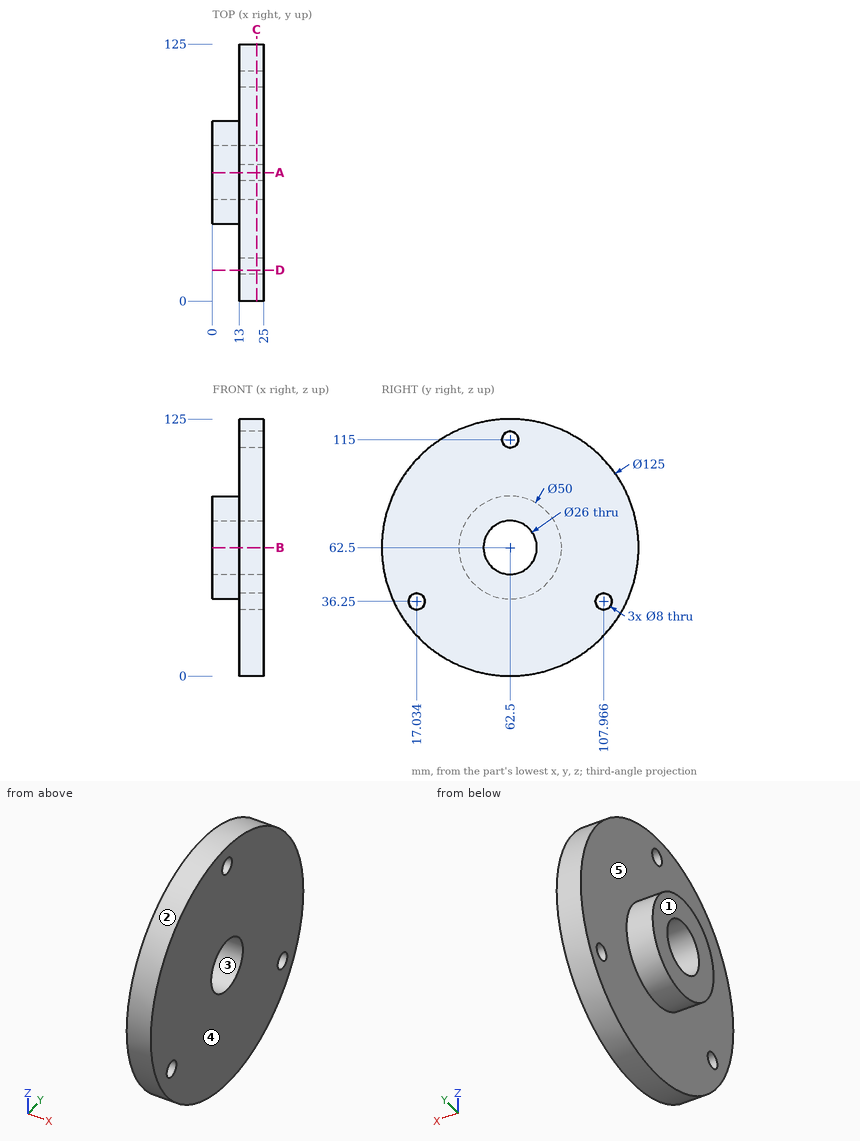
For this review, use the dimensioned drawing (mm, ordinates from the lowest corner) and the shaded views. A direction names the side the tool comes from. Give positions to 0.01 mm unless a question says otherwise; leave off trailing zeros. Loops run counter-clockwise (first coordinate to the right, second up) from the corner with the lowest first, then second, coordinate; pieces in that order, holes last.
Item 1: Tool access review of the marked faces 4 and 5: name each direction out of +Z, -Z, +X, -X, +Y, -Y from which nothing blocks a thin tool from reaching the whole face with its end or side.
Item 2: Insertion check: pin 1 (10.5 mm diameter, centred on y = 107.97, z = 36.25, fed in from +X); pin 2 (2 mm diameter, centred on x = 19.5, y = 81.5, fed in from +Z); pin 3 (10 mm diameter, centred on x = 10, y = 48.5, fed in from +Z) (1 decimal); pin 4 (1.5 mm diameter, centred on x = 6.5, z = 43, fed in from +Y) (1 decimal). Each pin has a flat end and moves straight along its axis. Give the tip position at first contact, or say it passes through.
Item 3: Take a section at A-A, the plane y = 62.5. State the section outline as (x, z) points, and give its area (3 significant figures).
Item 4: Take a section at C-C, the plane x = 21.5. State the section outline as (y, z) points.
Item 5: Take a section at D-D, the plane y = 15. State the section outline as (x, z) points (1 decimal).
Item 6: Take a section at B-B, the plane z = 62.5. State the section outline as (x, y) points.
Item 7: Draft analysis for pull direction Y (two halves, no side actions). For the marked faces 1, 2 and 3, state which applies: +Y half, -Y half, draft (parallel to the pull), parting line (faces both ways), or undercut.
Item 8: For line 1 along Y through (x, z) = (19, 36.25); line 2 along Z through (x, y) = (17.5, 62.5); line 3 along X through (y, z) = (23.5, 76.5), list the stretches that pass through material, from the lowest coordinate up.
Calculated:
1. face 4: +Z, -Z, +X, +Y, -Y
1. face 5: -X
2. pin 1: stops at x = 25
2. pin 2: stops at z = 122.35
2. pin 3: stops at z = 124.2
2. pin 4: stops at y = 79
3. outline: (0, 37.5) - (13, 37.5) - (13, 0) - (25, 0) - (25, 49.5) - (0, 49.5) - close; (0, 75.5) - (25, 75.5) - (25, 111) - (13, 111) - (13, 87.5) - (0, 87.5) - close; (13, 119) - (25, 119) - (25, 125) - (13, 125) - close
3. area: 1,400 mm2
4. outline: circle Ø125 at (62.5, 62.5); hole circle Ø8 at (17.03, 36.25); hole circle Ø26 at (62.5, 62.5); hole circle Ø8 at (62.5, 115); hole circle Ø8 at (107.97, 36.25)
5. outline: (13, 21.9) - (25, 21.9) - (25, 32.8) - (13, 32.8) - close; (13, 39.7) - (25, 39.7) - (25, 103.1) - (13, 103.1) - close
6. outline: (0, 37.5) - (13, 37.5) - (13, 0) - (25, 0) - (25, 49.5) - (0, 49.5) - close; (0, 75.5) - (25, 75.5) - (25, 125) - (13, 125) - (13, 87.5) - (0, 87.5) - close
7. face 1: draft
7. face 2: parting line
7. face 3: undercut
8. line 1: y = 5.78 to 13.03, 21.03 to 103.97, 111.97 to 119.22
8. line 2: z = 0 to 49.5, 75.5 to 111, 119 to 125
8. line 3: x = 13 to 25
